```python
from build123d import *

# Parameters (mm, degrees)
SKETCH1_W           = 75
SKETCH1_H           = 75
SKETCH1_R           = 2
SKETCH1_R_2         = 3.25
SKETCH1_R_3         = 1.75
BOSS_EXTRUDE1_DEPTH = 3


with BuildPart() as part:
    # Sketch1 → Boss-Extrude1 (new body)
    with BuildSketch(Plane(origin=(0, 0, 0), x_dir=(1, 0, 0), z_dir=(0, 1, 0))):
        Rectangle(SKETCH1_W, SKETCH1_H)
        with Locations((31.5, 31.5)):
            Circle(SKETCH1_R, mode=Mode.SUBTRACT)
        with Locations((31.5, -31.5)):
            Circle(SKETCH1_R, mode=Mode.SUBTRACT)
        with Locations((-31.5, -31.5)):
            Circle(SKETCH1_R, mode=Mode.SUBTRACT)
        with Locations((-31.5, 31.5)):
            Circle(SKETCH1_R, mode=Mode.SUBTRACT)
        with Locations((-22.5, 12.25)):
            Circle(SKETCH1_R_2, mode=Mode.SUBTRACT)
        with Locations((-7.5, 12.25)):
            Circle(SKETCH1_R_2, mode=Mode.SUBTRACT)
        with Locations((-24, 23.25)):
            Circle(SKETCH1_R_3, mode=Mode.SUBTRACT)
        with Locations((-6, 23.25)):
            Circle(SKETCH1_R_3, mode=Mode.SUBTRACT)
        with Locations((-24, 1.25)):
            Circle(SKETCH1_R_3, mode=Mode.SUBTRACT)
        with Locations((-6, 1.25)):
            Circle(SKETCH1_R_3, mode=Mode.SUBTRACT)
        with Locations((6, -22.5)):
            Circle(SKETCH1_R_3, mode=Mode.SUBTRACT)
        with Locations((24, -22.5)):
            Circle(SKETCH1_R_3, mode=Mode.SUBTRACT)
        with Locations((24, 2)):
            Circle(SKETCH1_R_3, mode=Mode.SUBTRACT)
        with Locations((6, 2)):
            Circle(SKETCH1_R_3, mode=Mode.SUBTRACT)
    extrude(amount=BOSS_EXTRUDE1_DEPTH)


solid = part.part
```
For this review, take the finished solid that the model builds, in its own axes (mm). Give positions to 0.01 mm unless a question says otherwise; leave off trailing zeros. Write each loop counter-clockwise with the first axis right and the second up, starting at its lowest first coordinate (ties: lowest second). Pieces come first, ordered by that corner, then holes.
Item 1: Wall thickness on probe 1 along Z at (x, y) = (31.5, 1.3); probe 2 along X at (y, z) = (1.1, -33); probe 3 along Z at (x, y) = (-7.5, 0.65): over which ranges is each line inside the solid? List them lowest first.
Item 2: Take a section at A-A (z = -23.25). Give the boundary of the cut face in (x, y), and give its area (3 significant figures).
Item 3: Take a section at D-D (x = -9). Give the boundary of the cut face in (y, z), and give its area (3 significant figures).
Item 4: Take a section at C-C (x = 24). Give the boundary of the cut face in (y, z).
Item 5: Take a section at B-B (y = 2.25). Give the number of separate pieces and of enclosed holes in the cut face, and give its area (3 significant figures).
Item 6: The part is to be moulded in two halves that separate along X. For faces 1 (the face through (-1, 0, -1)), 2 (the face through (-37.5, 1, 1)), 3 (the face through (-25.29, 1.48, -24.43)), say which applies: +X half, -X half, draft (parallel to the pull), parting line (faces both ways), or undercut.
Item 7: Insertion check: P1, Ø3, axis at x = -24, z = -23.25, coming from the +Y side; P2, Ø4.5, axis at x = -6, z = -1.25, coming from the -Y side. Each pin has a flat end and moves straight along its axis. Give the tip position at first contact, or say it passes through.
Established:
1. probe 1: z = -37.5 to -33.5, -29.5 to 29.5, 33.5 to 37.5
1. probe 2: x = -37.5 to -32.82, -30.18 to 30.18, 32.82 to 37.5
1. probe 3: z = -37.5 to -24.15, -22.35 to -15.5, -9 to -2.15, -0.35 to 37.5
2. outline: (-37.5, 0) - (-25.75, 0) - (-25.75, 3) - (-37.5, 3) - close; (-22.25, 0) - (-7.75, 0) - (-7.75, 3) - (-22.25, 3) - close; (-4.25, 0) - (37.5, 0) - (37.5, 3) - (-4.25, 3) - close
2. area: 204 mm2
3. outline: (0, -37.5) - (3, -37.5) - (3, -15.13) - (0, -15.13) - close; (0, -9.37) - (3, -9.37) - (3, 37.5) - (0, 37.5) - close
3. area: 208 mm2
4. outline: (0, -37.5) - (3, -37.5) - (3, -3.75) - (0, -3.75) - close; (0, -0.25) - (3, -0.25) - (3, 20.75) - (0, 20.75) - close; (0, 24.25) - (3, 24.25) - (3, 37.5) - (0, 37.5) - close
5. separate pieces: 1
5. enclosed holes: 14
5. area: 5,430 mm2
6. face 1: draft
6. face 2: -X half
6. face 3: undercut
7. P1: passes through
7. P2: stops at y = 0
